Source: CAD feature listing. Evaluate the final solid. Frame: model axes, mm. Face numbers are marked on the shaded views. A direction names the side the tool comes from. Give positions to 0.01 mm unless a question says otherwise; leave off trailing zeros. Loops run counter-clockwise (first coordinate to the right, second up) from the corner with the lowest first, then second, coordinate; pieces in that order, holes last. Notation, with made-up numbers: M 60.25,37 L 66.25,37 A29 cw 66.25,71 Z; hole C -11,50 d2. An arc over 180 degrees is marked long. Write item = value, one per line.
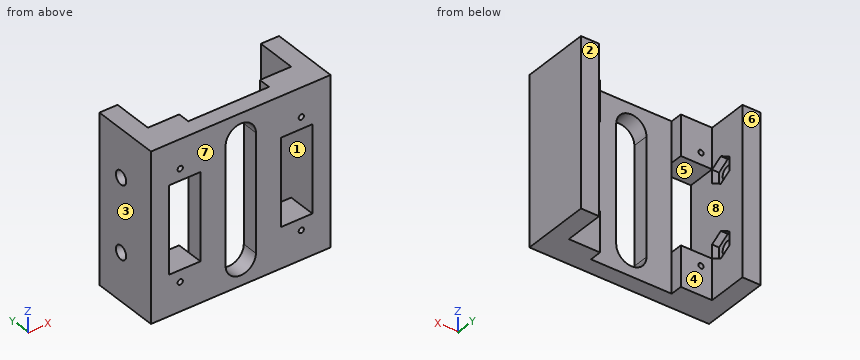
from build123d import *

# Parameters (mm, degrees)
SKETCH1_W                = 89
SKETCH1_H                = 83
SKETCH1_R                = 1.3
MAIN_BODY_DEPTH          = 14
SKETCH2_W                = 40
SKETCH2_H                = 83
SCREW_GROOVE_DEPTH       = 6
SKETCH4_W                = 9
SKETCH4_H                = 83
MOUNT_LIFT_DEPTH         = 20
MOUNT_START              = -5.55625
MOUNT_NUTS_DEPTH         = 18.94375
F_9_32_MOUNT_HOLES_REACH = 7.556
SKETCH5_R                = 3.3734375
SKETCH8_W                = 15.5
SKETCH8_H                = 43
MIDDLE_CUT_DEPTH         = 14


with BuildPart() as part:
    # Sketch1 → Main Body (new body)
    with BuildSketch(Plane(origin=(0, 0, 0), x_dir=(1, 0, 0), z_dir=(0, 1, 0))):
        with Locations((0, 41.5)):
            Rectangle(SKETCH1_W, SKETCH1_H)
        with Locations((-30, 14.25)):
            Circle(SKETCH1_R, mode=Mode.SUBTRACT)
        with Locations((30, 14.25)):
            Circle(SKETCH1_R, mode=Mode.SUBTRACT)
        with BuildLine():
            Line((-7.5, 12.5), (-7.5, 70.5))
            ThreePointArc((-7.5, 70.5), (0, 78), (7.5, 70.5))
            Line((7.5, 70.5), (7.5, 12.5))
            ThreePointArc((7.5, 12.5), (0, 5), (-7.5, 12.5))
        make_face(mode=Mode.SUBTRACT)
        with Locations((-30, 68.75)):
            Circle(SKETCH1_R, mode=Mode.SUBTRACT)
        with Locations((30, 68.75)):
            Circle(SKETCH1_R, mode=Mode.SUBTRACT)
    extrude(amount=MAIN_BODY_DEPTH)

    # Sketch2 → Screw Groove (cut)
    with BuildSketch(Plane(origin=(0, 14, 0), x_dir=(1, 0, 0), z_dir=(0, 1, 0))):
        with Locations((0, 41.5)):
            Rectangle(SKETCH2_W, SKETCH2_H)
    extrude(amount=-SCREW_GROOVE_DEPTH, mode=Mode.SUBTRACT)

    # Sketch4 → Mount Lift (add)
    with BuildSketch(Plane(origin=(0, 14, 0), x_dir=(1, 0, 0), z_dir=(0, 1, 0))):
        with Locations((-40, 41.5)):
            Rectangle(SKETCH4_W, SKETCH4_H)
        with Locations((40, 41.5)):
            Rectangle(SKETCH4_W, SKETCH4_H)
    extrude(amount=MOUNT_LIFT_DEPTH)

    # Sketch6 → Mount Nuts (cut)
    with BuildSketch(Plane.ZY.offset(44.5).offset(MOUNT_START)):
        Polygon((-52.855059246, 19.7546875), (-56.177529623, 25.509375), (-62.822470377, 25.509375), (-66.144940754, 19.7546875), (-62.822470377, 14), (-56.177529623, 14), align=None)
        Polygon((-16.855059246, 19.7546875), (-20.177529623, 25.509375), (-26.822470377, 25.509375), (-30.144940754, 19.7546875), (-26.822470377, 14), (-20.177529623, 14), align=None)
    extrude(amount=-MOUNT_NUTS_DEPTH, mode=Mode.SUBTRACT)

    # Sketch5 → 9/32 Mount Holes (cut, up to next)
    with BuildSketch(Plane.ZY.offset(38.94375), mode=Mode.PRIVATE) as f_9_32_mount_holes_sk1:
        with Locations((-59.5, 19.7546875)):
            Circle(SKETCH5_R)
    f_9_32_mount_holes_tool1 = extrude(f_9_32_mount_holes_sk1.sketch, amount=F_9_32_MOUNT_HOLES_REACH, mode=Mode.PRIVATE) & part.part
    add(f_9_32_mount_holes_tool1.solids().sort_by_distance((-38.94375, 19.754688, -59.5))[0], mode=Mode.SUBTRACT)
    # Sketch5 → 9/32 Mount Holes (cut, up to next)
    with BuildSketch(Plane.ZY.offset(38.94375), mode=Mode.PRIVATE) as f_9_32_mount_holes_sk2:
        with Locations((-23.5, 19.7546875)):
            Circle(SKETCH5_R)
    f_9_32_mount_holes_tool2 = extrude(f_9_32_mount_holes_sk2.sketch, amount=F_9_32_MOUNT_HOLES_REACH, mode=Mode.PRIVATE) & part.part
    add(f_9_32_mount_holes_tool2.solids().sort_by_distance((-38.94375, 19.754688, -23.5))[0], mode=Mode.SUBTRACT)

    # Sketch8 → Middle Cut (cut)
    with BuildSketch(Plane(origin=(0, 14, 0), x_dir=(1, 0, 0), z_dir=(0, 1, 0))):
        with Locations((-27.75, 41.5)):
            Rectangle(SKETCH8_W, SKETCH8_H)
        with Locations((27.75, 41.5)):
            Rectangle(SKETCH8_W, SKETCH8_H)
    extrude(amount=-MIDDLE_CUT_DEPTH, mode=Mode.SUBTRACT)


solid = part.part
1. Pull-direction query (X, two-part tool) for the marked faces 1, 2 and 3; classes: +X half, -X half, draft (parallel to the pull), parting line (faces both ways), or undercut.
Derived:
face_1 = undercut
face_2 = draft
face_3 = -X half
2. Cut plane D-D, the plane y = 28.5. Return the cut outline in (x, z), then the cut area to 3 significant figures.
Derived:
outline = M -44.5,-83 L -35.5,-83 L -35.5,0 L -44.5,0 Z; M 35.5,-83 L 44.5,-83 L 44.5,0 L 35.5,0 Z
area = 1,490 mm²
3. Reachability of the marked faces 4, 5, 6, 7 and 8 from +Z, -Z, +X, -X, +Y, -Y: full face, straight path, thin tool, end or side. Return the list, or none.
Derived:
face_4 = +Z, -Z, +Y
face_5 = +Y, -Y
face_6 = +Z, -Z, +X, -X, +Y
face_7 = +Z, -Z, +X, -X, -Y
face_8 = +Y
4. Cut plane A-A, the plane y = 11. Return the cut outline in (x, z), then the cut area to 3 significant figures.
Derived:
outline = M -44.5,-83 L -20,-83 L -20,-63 L -35.5,-63 L -35.5,-20 L -20,-20 L -20,0 L -44.5,0 Z; M 20,-83 L 44.5,-83 L 44.5,0 L 20,0 L 20,-20 L 35.5,-20 L 35.5,-63 L 20,-63 Z; hole C -30,-68.75 d2.6; hole C -30,-14.25 d2.6; hole C 30,-68.75 d2.6; hole C 30,-14.25 d2.6
area = 2,710 mm²
5. First-contact query: pin 1 Ø1.5 at (x, z) = (-14, -19.5) entering from +Y; pin 2 Ø2 at (x, z) = (-30, -14.25) entering from +Y; pin 3 Ø5 at (x, z) = (25.5, -70.5) entering from +Y. Flat tips, straight axial feed; report the tip coordinate or a pass-through.
Derived:
pin_1 = 8
pin_2 = through
pin_3 = 14
6. Cut plane C-C, the plane x = -21.5. Return the cut outline in (y, z), then the cut area to 3 significant figures.
Derived:
outline = M 0,-83 L 14,-83 L 14,-63 L 0,-63 Z; M 0,-20 L 14,-20 L 14,0 L 0,0 Z
area = 560 mm²
7. Cut plane B-B, the plane z = -51.5. Return the cut outline in (x, y), then the cut area to 3 significant figures.
Derived:
outline = M -44.5,0 L -35.5,0 L -35.5,34 L -44.5,34 Z; M -20,0 L -7.5,0 L -7.5,8 L -20,8 Z; M 7.5,0 L 20,0 L 20,8 L 7.5,8 Z; M 35.5,0 L 44.5,0 L 44.5,34 L 35.5,34 Z
area = 812 mm²
8. Material intervals for probe 1 along X at (y, z) = (1, -25); probe 2 along X at (y, z) = (3, -68.75); probe 3 along Y at (x, z) = (-42.35, -23.5), sorted ascending. Write a range as from..to.
Derived:
probe_1 = -44.5..-35.5, -20..-7.5, 7.5..20, 35.5..44.5
probe_2 = -44.5..-31.3, -28.7..-7.5, 7.5..28.7, 31.3..44.5
probe_3 = 0..16.38, 23.13..34
